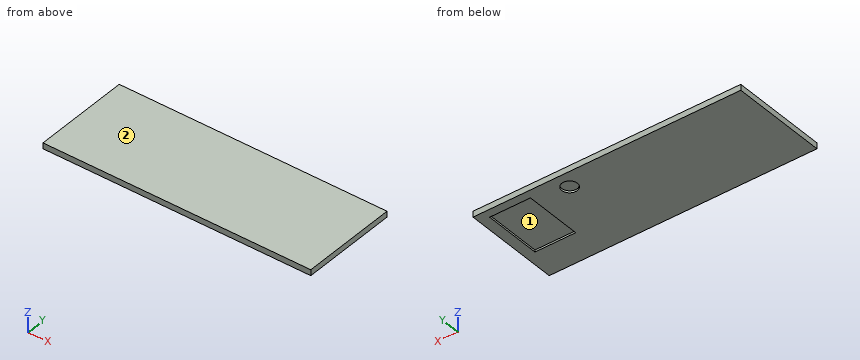
from build123d import *

# Parameters (mm, degrees)
CROQUIS1_W              = 1380
CROQUIS1_H              = 500
SALIENTE_EXTRUIR1_DEPTH = 30
CROQUIS2_R              = 40
CROQUIS2_W              = 210
CROQUIS2_H              = 297
CORTAR_EXTRUIR3_DEPTH   = 10


with BuildPart() as part:
    # Croquis1 → Saliente-Extruir1 (new body)
    with BuildSketch(Plane.XY):
        Rectangle(CROQUIS1_W, CROQUIS1_H)
    extrude(amount=SALIENTE_EXTRUIR1_DEPTH)

    # Croquis2 → Cortar-Extruir3 (cut)
    with BuildSketch(Plane(origin=(0, 0, 0), x_dir=(-1, 0, 0), z_dir=(0, 0, -1))):
        with Locations((-256.532724235, 167.997980694)):
            Circle(CROQUIS2_R)
        with Locations((-532.122165127, 59.369001894)):
            Rectangle(CROQUIS2_W, CROQUIS2_H)
    extrude(amount=-CORTAR_EXTRUIR3_DEPTH, mode=Mode.SUBTRACT)


solid = part.part
Verification items for the finished model (mm, model axes). Face numbers are marked on the shaded views. Coordinates: 2 decimals unless noted, no trailing zeros. Write each loop counter-clockwise with the first axis right and the second up, starting at its lowest first coordinate (ties: lowest second). Pieces come first, ordered by that corner, then holes. Notation, with made-up numbers: M 2.25,9 L 36.25,9 A11 ccw 36.25,22 Z; hole C 20.25,42.25 d3. An arc over 180 degrees is marked long. Use a Markdown table: item, result.
Q1. Sectioned sample at B-B, the plane z = 5. Record the boundary of the cut face in (x, y), plus the area to 3 significant figures.
Reply:
| item | result |
|---|---|
| outline | M -690,-250 L 690,-250 L 690,250 L -690,250 Z; hole C 256.53,168 d80; hole M 427.12,-89.13 L 637.12,-89.13 L 637.12,207.87 L 427.12,207.87 Z |
| area | 623,000 mm² |
Q2. Sectioned sample at A-A, the plane y = 73. Record the boundary of the cut face in (x, z).
Reply:
| item | result |
|---|---|
| outline | M -690,0 L 427.12,0 L 427.12,10 L 637.12,10 L 637.12,0 L 690,0 L 690,30 L -690,30 Z |
Q3. Thickness scan on line 1 (X direction, y = -11, z = 1.5); line 2 (Z direction, x = 427.5, y = 151). Record the ranges inside material, lowest first.
Reply:
| item | result |
|---|---|
| line 1 | x = -690 to 427.12, 637.12 to 690 |
| line 2 | z = 10 to 30 |
Q4. Draft check along X on the marked faces 1 and 2. Enter one of: +X half, -X half, draft (parallel to the pull), parting line (faces both ways), or undercut.
Reply:
| item | result |
|---|---|
| face 1 | undercut |
| face 2 | draft |
